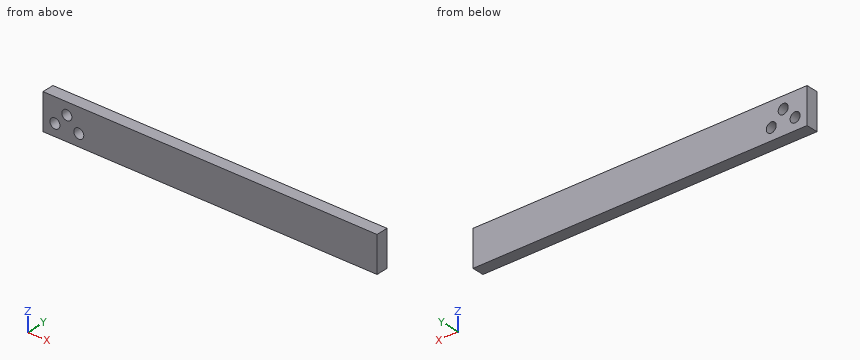
```python
from build123d import *

# Parameters (mm, degrees)
SKETCH1_W                      = 177.8
SKETCH1_H                      = 19.05
BOSS_EXTRUDE1_DEPTH            = 6.35
F_4_0_209_DIAMETER_HOLE1_D     = 5.3086
F_4_0_209_DIAMETER_HOLE1_DEPTH = 10.668
F_4_0_209_DIAMETER_HOLE1_TIP   = 1.594864341


with BuildPart() as part:
    # Sketch1 → Boss-Extrude1 (new body)
    with BuildSketch(Plane(origin=(0, 0, 0), x_dir=(1, 0, 0), z_dir=(0, 1, 0))):
        with Locations((88.9, 9.525)):
            Rectangle(SKETCH1_W, SKETCH1_H)
    extrude(amount=BOSS_EXTRUDE1_DEPTH)

    # #4 (0.209) Diameter Hole1
    with Locations(Plane(origin=(6.35, 6.35, -12.7), x_dir=(0, 0, 1), z_dir=(0, 1, 0))):
        with Locations((0, 0), (0, 12.7), (6.35, 6.35)):
            Hole(F_4_0_209_DIAMETER_HOLE1_D / 2, depth=F_4_0_209_DIAMETER_HOLE1_DEPTH)
            with Locations((0, 0, -(F_4_0_209_DIAMETER_HOLE1_DEPTH + F_4_0_209_DIAMETER_HOLE1_TIP / 2))):  # 118° drill point
                Cone(0, F_4_0_209_DIAMETER_HOLE1_D / 2, F_4_0_209_DIAMETER_HOLE1_TIP, mode=Mode.SUBTRACT)


solid = part.part
```
Input: part model. Units: mm. Frame: model coordinates. Coordinates: 2 decimals unless noted, no trailing zeros. Write each loop counter-clockwise with the first axis right and the second up, starting at its lowest first coordinate (ties: lowest second). Pieces come first, ordered by that corner, then holes. Notation, with made-up numbers: (26.5, 17) - (80.5, 17) arc R28 cw to (80.5, 39) - close; hole circle Ø1 at (65, -7.75). An arc over 180 degrees is marked (long way). Put each result on its own line as item: value. Start each with the question number.
1) Cut plane B-B (x = 12.7). Return the cut outline in (y, z).
2) Cut plane C-C (y = 1.5). Return the cut outline in (x, z), plus the area to 3 significant figures.
3) Contact query for a flat-ended pin moving along its axis: pin 1 (4 mm diameter, centred on x = 51.5, z = -4, fed in from -Y). Output: stop coordinate, or through.
4) Ray query, L1, parallel to X at y = 4.5, z = -13; L2, parallel to X at y = 2, z = -6.25; L3, parallel to X at y = 0.5, z = -8.25. Return the intervals inside material, ascending.
5) Cut plane D-D (z = -6.35). Return the cut outline in (x, y).
6) Cut plane A-A (z = -12.7). Return the cut outline in (x, y), plus the area to 3 significant figures.
Resolved:
1. outline: (0, -19.05) - (6.35, -19.05) - (6.35, -9) - (0, -9) - close; (0, -3.7) - (6.35, -3.7) - (6.35, 0) - (0, 0) - close
2. outline: (0, -19.05) - (177.8, -19.05) - (177.8, 0) - (0, 0) - close; hole circle Ø5.31 at (6.35, -12.7); hole circle Ø5.31 at (12.7, -6.35); hole circle Ø5.31 at (19.05, -12.7)
2. area: 3,320 mm2
3. pin 1: stops at y = 0
4. L1: x = 0 to 3.71, 8.99 to 16.41, 21.69 to 177.8
4. L2: x = 0 to 10.05, 15.35 to 177.8
4. L3: x = 0 to 10.85, 14.55 to 177.8
5. outline: (0, 0) - (10.05, 0) - (10.05, 6.35) - (0, 6.35) - close; (15.35, 0) - (177.8, 0) - (177.8, 6.35) - (15.35, 6.35) - close
6. outline: (0, 0) - (3.7, 0) - (3.7, 6.35) - (0, 6.35) - close; (9, 0) - (16.4, 0) - (16.4, 6.35) - (9, 6.35) - close; (21.7, 0) - (177.8, 0) - (177.8, 6.35) - (21.7, 6.35) - close
6. area: 1,060 mm2
